```python
from build123d import *

# Parameters (mm, degrees)
SKETCH1_W           = 88.9
SKETCH1_H           = 82.55
BOSS_EXTRUDE1_DEPTH = 6.35
SKETCH2_R           = 12.7
SKETCH2_W           = 12.7
SKETCH2_H           = 6.35
SKETCH2_W_2         = 6.35
SKETCH2_H_2         = 25.4
SKETCH2_H_3         = 12.7
CUT_EXTRUDE2_DEPTH  = 6.35


with BuildPart() as part:
    # Sketch1 → Boss-Extrude1 (new body)
    with BuildSketch(Plane.YZ):
        with Locations((44.45, 41.275)):
            Rectangle(SKETCH1_W, SKETCH1_H)
    extrude(amount=BOSS_EXTRUDE1_DEPTH)

    # Sketch2 → Cut-Extrude2 (cut)
    with BuildSketch(Plane.YZ.offset(6.35)):
        with Locations((44.45, 82.55)):
            Circle(SKETCH2_R)
        with Locations((57.15, 3.175)):
            Rectangle(SKETCH2_W, SKETCH2_H)
        with Locations((31.75, 3.175)):
            Rectangle(SKETCH2_W, SKETCH2_H)
        Polygon((0, 0), (12.7, 0), (12.7, 6.35), (6.35, 6.35), (6.35, 19.05), (0, 19.05), (0, 6.35), align=None)
        Polygon((76.2, 0), (88.9, 0), (88.9, 6.35), (88.9, 19.05), (82.55, 19.05), (82.55, 6.35), (76.2, 6.35), align=None)
        with Locations((3.175, 69.85)):
            Rectangle(SKETCH2_W_2, SKETCH2_H_2)
        with Locations((3.175, 38.1)):
            Rectangle(SKETCH2_W_2, SKETCH2_H_3)
        with Locations((85.725, 38.1)):
            Rectangle(SKETCH2_W_2, SKETCH2_H_3)
        with Locations((85.725, 69.85)):
            Rectangle(SKETCH2_W_2, SKETCH2_H_2)
    extrude(amount=-CUT_EXTRUDE2_DEPTH, mode=Mode.SUBTRACT)


solid = part.part
```
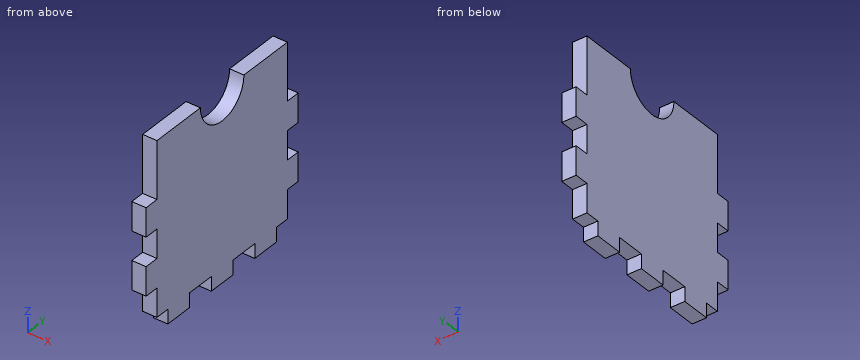
Check sheet for the modelled part. Datum: model origin and axes. Units: mm. Round coordinates to 2 decimals unless told otherwise and drop trailing zeros. Order: outer loops, then holes, each group sorted by start corner. A loop starts at its lowest first (then second) coordinate and runs counter-clockwise, first axis right, second up. Notation, with made-up numbers: (-2.5, -11) -> (56.5, -11) arc R11 ccw to (56.5, 5) -> close; hole circle Ø10 at (-24, -17.5). An arc over 180 degrees is marked (long way). Use CSV: the item, a comma, the result in double quotes.
(1) Material ranges on line 1 along Y through (x, z) = (5, 5); line 2 along Y through (x, z) = (1.5, 18.5); line 3 along Z through (x, y) = (0.75, 85), recorded low to high. Write a range as from..to.
Worked out:
line 1,"12.7..25.4, 38.1..50.8, 63.5..76.2"
line 2,"6.35..82.55"
line 3,"19.05..31.75, 44.45..57.15"
(2) Depth check by flat-ended pin: pin 1 (3 mm diameter, centred on x = 3, y = 87, fed in from -Z); pin 2 (1.9 mm diameter, centred on x = 3.5, z = 35, fed in from -Y); pin 3 (3 mm diameter, centred on x = 3, z = 64.5, fed in from +Y). Enter the tip coordinate at first touch or a pass-through.
Worked out:
pin 1,"z = 19.05"
pin 2,"y = 6.35"
pin 3,"y = 82.55"
(3) Cross-section at B-B (z = 61). Record the boundary of the cut face in (x, y), and give its area (3 significant figures).
Worked out:
outline,"(0, 6.35) -> (6.35, 6.35) -> (6.35, 82.55) -> (0, 82.55) -> close"
area,"484 mm²"
